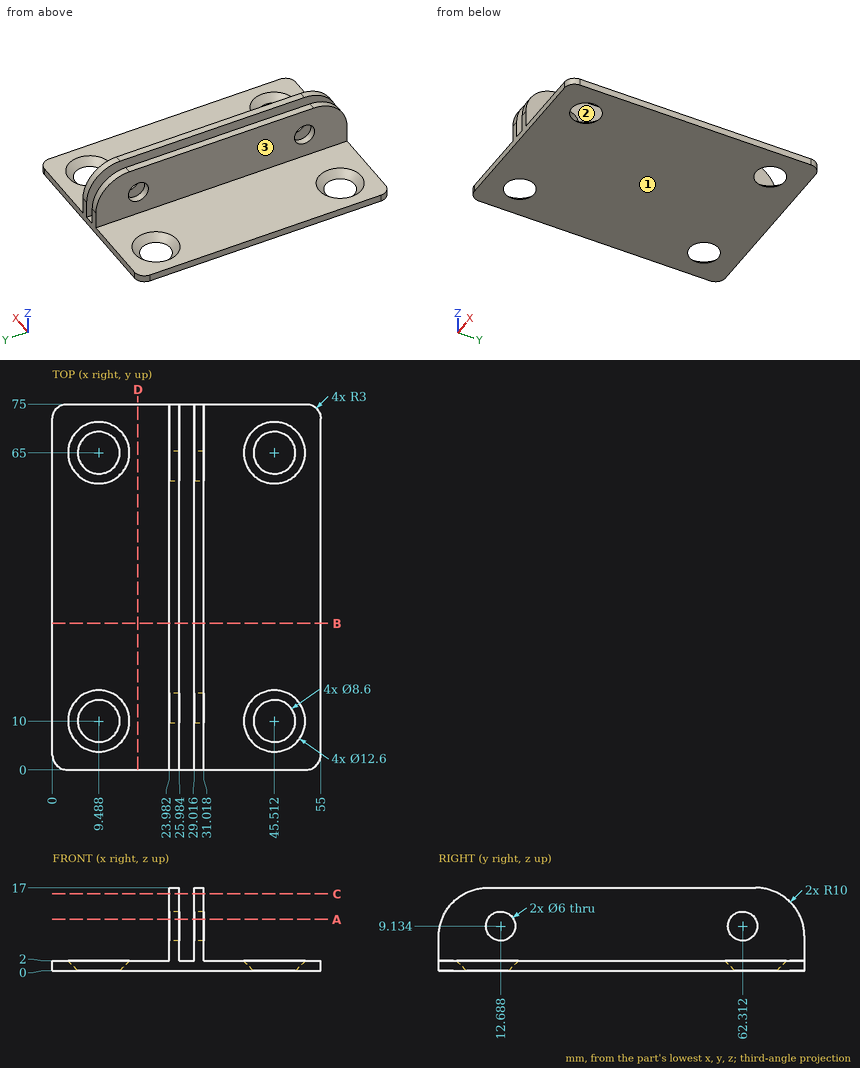
Answer from the drawing. Dimensions are ordinates in mm from the lowest x, y and z of the part. A direction names the side the tool comes from. Give positions to 0.01 mm unless a question says otherwise; leave off trailing zeros. Loops run counter-clockwise (first coordinate to the right, second up) from the corner with the lowest first, then second, coordinate; pieces in that order, holes last. Notation, with made-up numbers: M -24,23 L -19,23 A18 ccw -19,40 Z; hole C 24,86 d8. An arc over 180 degrees is marked long. One line per item, written item: value.
Q1. Flat-ended cylindrical pins translate along their axes: P1, Ø9.5, axis at y = 12.69, z = 9.13, coming from the +X side; P2, Ø7, axis at x = 38.5, y = 30.5, coming from the +Z side; P3, Ø6, axis at y = 51.5, z = 5.5, coming from the -X side. Find the tip coordinate at first contact, or state that the pin passes through.
Working result:
P1: stops at x = 31.02
P2: stops at z = 2
P3: stops at x = 23.98
Q2. A cutting plane is placed at C-C on z = 15.75. Determine the outline of the cut face in (x, y), then the cut area to 3 significant figures.
Working result:
outline: M 23.98,5.16 L 25.98,5.16 L 25.98,69.84 L 23.98,69.84 Z; M 29.02,5.16 L 31.02,5.16 L 31.02,69.84 L 29.02,69.84 Z
area: 259 mm^2
Q3. A cutting plane is placed at B-B on y = 30. Determine the outline of the cut face in (x, z).
Working result:
outline: M 0,0 L 55,0 L 55,2 L 31.02,2 L 31.02,17 L 29.02,17 L 29.02,2 L 25.98,2 L 25.98,17 L 23.98,17 L 23.98,2 L 0,2 Z
Q4. A cutting plane is placed at D-D on x = 17.5. Determine the outline of the cut face in (y, z), then the cut area to 3 significant figures.
Working result:
outline: M 0,0 L 75,0 L 75,2 L 0,2 Z
area: 150 mm^2
Q5. For the marked faces 1, 2 and 3, determine the directions among +Z, -Z, +X, -X, +Y, -Y from which every point of the face is accessible in a straight line to the end or side of a thin tool.
Working result:
face 1: -Z, +X, -X, +Y, -Y
face 2: +Z, +X, +Y, -Y
face 3: +Z, -X, +Y, -Y
Q6. Find the intervals of material crossed by line 1 (X direction, y = 70.5, z = 6.5); line 2 (Z direction, x = 11.5, y = 72.5); line 3 (Z direction, x = 24.5, y = 71), in increasing order. Write a range as from..to.
Working result:
line 1: x = 23.98..25.98, 29.02..31.02
line 2: z = 0..2
line 3: z = 0..15
Q7. A cutting plane is placed at A-A on z = 10.5. Determine the outline of the cut face in (x, y).
Working result:
outline: M 23.98,0.63 L 25.98,0.63 L 25.98,10.02 L 23.98,10.02 Z; M 23.98,15.36 L 25.98,15.36 L 25.98,59.64 L 23.98,59.64 Z; M 23.98,64.98 L 25.98,64.98 L 25.98,74.37 L 23.98,74.37 Z; M 29.02,0.63 L 31.02,0.63 L 31.02,10.02 L 29.02,10.02 Z; M 29.02,15.36 L 31.02,15.36 L 31.02,59.64 L 29.02,59.64 Z; M 29.02,64.98 L 31.02,64.98 L 31.02,74.37 L 29.02,74.37 Z
